Part model, mm, in its own coordinate system. Face numbers are marked on the shaded views. A direction names the side the tool comes from. Coordinates: 2 decimals unless noted, no trailing zeros. Loops run counter-clockwise (first coordinate to the right, second up) from the corner with the lowest first, then second, coordinate; pieces in that order, holes last. Notation, with made-up numbers: M 61.5,52.5 L 120.5,52.5 A25 cw 120.5,70.5 Z; hole C -27.5,-20 d4. An arc over 180 degrees is marked long. Use a Markdown table: item, result. Add a question column.
1) Band-saw the part on A-A (z = 4). List the corners of the cut face in (x, y), plus the area to 3 significant figures.
2) Wall check: probe 1 along Y at (x, z) = (0, 4.25); probe 2 along Z at (x, y) = (6.75, -5); probe 3 along Z at (x, y) = (-3.5, 1.75). Give the ranges that are in metal, low to high. Write a range as from..to.
3) Pin check, flat tips, straight feed: pin 1 Ø2.5 at (y, z) = (-2, 5.5) entering from +X; pin 2 Ø3 at (x, y) = (6.5, -6.5) entering from +Z; pin 3 Ø1 at (x, z) = (4, 3) entering from -Y. Stop position of each tip, or through.
4) Band-saw the part on D-D (z = -0.25). List the corners of the cut face in (x, y), plus the area to 4 significant figures.
5) Band-saw the part on B-B (x = -0.5). List the corners of the cut face in (y, z).
6) Tool access for the marked faces 1, 2, 3 and 4: list every direction of +Z, -Z, +X, -X, +Y, -Y with a clear straight run to the whole face (end or side of a thin tool).
7) Band-saw the part on C-C (y = -4.75). List the corners of the cut face in (x, z), plus the area to 3 significant figures.
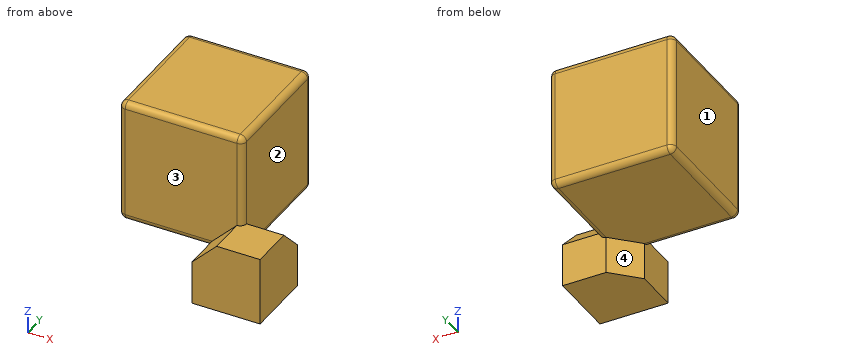
from build123d import *

# Parameters (mm, degrees)
SKETCH1_W                = 10
SKETCH1_H                = 10
BASE_EXTRUDE_DEPTH       = 10
BOSS_EXTRUDE1_DEPTH      = 5
BOSS_EXTRUDE1_DEPTH_BACK = 0.5
SKETCH3_W                = 5.5
SKETCH3_H                = 5.5
FILLET2_R                = 0.5
CHAMFER4_SIZE            = 2


with BuildPart() as part:
    # Sketch1 → Base-Extrude (new body)
    with BuildSketch(Plane.XY):
        Rectangle(SKETCH1_W, SKETCH1_H)
    extrude(amount=BASE_EXTRUDE_DEPTH)

    # Sketch3 → Boss-Extrude1 (add, two sides: drawn at the far end of the back side and taken through both)
    with BuildSketch(Plane(origin=(3, 0, 0), x_dir=(0, 0, -1), z_dir=(1, 0, 0)).offset(-BOSS_EXTRUDE1_DEPTH_BACK)):
        with Locations((0.25, -5.25)):
            Rectangle(SKETCH3_W, SKETCH3_H)
    extrude(amount=BOSS_EXTRUDE1_DEPTH + BOSS_EXTRUDE1_DEPTH_BACK)

    # Fillet2
    fillet2_edges = [part.edges().sort_by_distance(p)[0] for p in [
        (-5, 5, 5),
        (5, 5, 5),
        (0, 5, 0),
        (0, 5, 10),
        (-5, -5, 5),
        (-5, 0, 0),
        (-5, 0, 10),
        (5, 1.25, 0),
        (5, -5, 6.25),
        (5, 0, 10),
        (-1.25, -5, 0),
        (0, -5, 10),
    ]]
    fillet(fillet2_edges, radius=FILLET2_R)

    # Chamfer4
    chamfer4_edges = [part.edges().sort_by_distance(p)[0] for p in [
        (2.5, -2.5, -1.5),
        (2.5, -6.5, 2.5),
        (6.5, -2.5, 2.5),
    ]]
    chamfer(chamfer4_edges, length=CHAMFER4_SIZE)


solid = part.part
Entries:
| question | item | result |
|---|---|---|
| 1 | outline | M -5,-4.5 A0.5 ccw -4.5,-5 L 4.5,-5 A0.5 ccw 5,-4.5 L 5,4.5 A0.5 ccw 4.5,5 L -4.5,5 A0.5 ccw -5,4.5 Z |
| 1 | area | 99.8 mm2 |
| 2 | probe 1 | -5..5 |
| 2 | probe 2 | -3..2.5 |
| 2 | probe 3 | 0..10 |
| 3 | pin 1 | x = 5 |
| 3 | pin 2 | z = 2.5 |
| 3 | pin 3 | y = -5 |
| 4 | outline | M 2.5,-8 L 8,-8 L 8,-2.5 L 4.5,-2.5 L 2.5,-4.5 Z |
| 4 | area | 28.25 mm2 |
| 5 | outline | M -5,0.5 A0.5 ccw -4.5,0 L 4.5,0 A0.5 ccw 5,0.5 L 5,9.5 A0.5 ccw 4.5,10 L -4.5,10 A0.5 ccw -5,9.5 Z |
| 6 | face 1 | +Z, -Z, -X, +Y, -Y |
| 6 | face 2 | +Z, +X, +Y |
| 6 | face 3 | +Z, -X, -Y |
| 6 | face 4 | -Z, -X, +Y |
| 7 | outline | M -4.93,0.5 A0.43 ccw -4.5,0.07 L 2.5,0.07 L 2.5,-3 L 8,-3 L 8,2.5 L 4.93,2.5 L 4.93,9.5 A0.43 ccw 4.5,9.93 L -4.5,9.93 A0.43 ccw -4.93,9.5 Z |
| 7 | area | 122 mm2 |
